Autodesk Inventor part; units mm, degrees
ref_plane "YZ Plane" through (0, 0, 0) normal (1, 0, 0) x (0, 1, 0)
ref_plane "XZ Plane" through (0, 0, 0) normal (0, 1, 0) x (-1, 0, 0)
ref_plane "XY Plane" through (0, 0, 0) normal (0, 0, 1) x (1, 0, 0)
sketch "Эскиз1" plane through (0, 0, 0) normal (0, 1, 0) x (-1, 0, 0)
  circle A0 centre (0, 0) radius 9.5
  circle A1 centre (0, 0) radius 25
  circle A2 centre (14, 0) radius 2
  circle A3 centre (4.3262, 13.3148) radius 2
  circle A4 centre (-11.3262, 8.229) radius 2
  circle A5 centre (-11.3262, -8.229) radius 2
  circle A6 centre (4.3262, -13.3148) radius 2
  dimension "d0" = 19
  dimension "d1" = 50
  dimension "d2" = 4
  dimension "d3" = 14
  dimension "d6" = 360
extrude "Выдавливание1" add sketch "Эскиз1" along normal blind 5
properties part number "ротор мотора"
Work out the finished part from the listing and answer in its coordinate system (mm). Round coordinates to 2 decimals unless told otherwise and drop trailing zeros. Write each loop counter-clockwise with the first axis right and the second up, starting at its lowest first coordinate (ties: lowest second). Pieces come first, ordered by that corner, then holes. Notation, with made-up numbers: (48, 57) - (59, 57) arc R11 cw to (59, 71) - close; hole circle Ø8 at (53.25, -13.75). An arc over 180 degrees is marked (long way). Answer in a Markdown table with one row per item. Add a question column.
1. Find the intervals of material crossed by line 1 along Z through (x, y) = (0, 2.2); line 2 along X through (y, z) = (2.6, -1.5); line 3 along Z through (x, y) = (-14.5, 4.2), in increasing order. Write a range as from..to.
2. Given pin 1 (2.5 mm diameter, centred on x = -14, z = 0, fed in from -Y); pin 2 (1.5 mm diameter, centred on x = 4, y = 3, fed in from +Z); pin 3 (2 mm diameter, centred on x = -12.5, y = 2, fed in from -Z); pin 4 (2 mm diameter, centred on y = 1.5, z = 19, fed in from +X), each flat-ended and moving along its own axis, determine where each tip first touches the part or whether it passes through.
3. A cutting plane is placed at C-C, the plane z = 5. Determine the outline of the cut face in (x, y), and give its area (3 significant figures).
4. A cutting plane is placed at D-D, the plane y = 1.2. Determine the outline of the cut face in (x, z).
5. The mould has two halves that part along X. Classify faces 1 (the flat face through (0, 5, -11)), 2 (the cylindrical face through (-12.4, 2.5, 1.2)), 3 (the cylindrical face through (-23.846, 2.465, -7.509)): +X half, -X half, draft (parallel to the pull), parting line (faces both ways), or undercut.
6. A cutting plane is placed at A-A, the plane z = 0. Determine the outline of the cut face in (x, y).
7. A cutting plane is placed at B-B, the plane x = 0. Determine the outline of the cut face in (y, z), and give its area (3 significant figures).
Worked out:
| question | item | result |
|---|---|---|
| 1 | line 1 | -25..-9.5, 9.5..25 |
| 1 | line 2 | -24.95..-15.32, -12.68..-9.38, 9.38..24.95 |
| 1 | line 3 | -20.37..-1.94, 1.94..20.37 |
| 2 | pin 1 | through |
| 2 | pin 2 | z = 24.79 |
| 2 | pin 3 | z = -22.2 |
| 2 | pin 4 | x = 17.35 |
| 3 | outline | (-24.49, 0) - (-8.08, 0) - (-8.08, 5) - (-24.49, 5) - close; (8.08, 0) - (24.49, 0) - (24.49, 5) - (8.08, 5) - close |
| 3 | area | 164 mm^2 |
| 4 | outline | circle Ø50 at (0, 0); hole circle Ø4 at (-14, 0); hole circle Ø19 at (0, 0); hole circle Ø4 at (-4.33, -13.31); hole circle Ø4 at (-4.33, 13.31); hole circle Ø4 at (11.33, -8.23); hole circle Ø4 at (11.33, 8.23) |
| 5 | face 1 | draft |
| 5 | face 2 | undercut |
| 5 | face 3 | parting line |
| 6 | outline | (-25, 0) - (-16, 0) - (-16, 5) - (-25, 5) - close; (-12, 0) - (-9.5, 0) - (-9.5, 5) - (-12, 5) - close; (9.5, 0) - (25, 0) - (25, 5) - (9.5, 5) - close |
| 7 | outline | (0, -25) - (5, -25) - (5, -9.5) - (0, -9.5) - close; (0, 9.5) - (5, 9.5) - (5, 25) - (0, 25) - close |
| 7 | area | 155 mm^2 |
